Geometry: final body of the model. Coordinates: model frame, mm. A direction names the side the tool comes from. Give positions to 0.01 mm unless a question says otherwise; leave off trailing zeros. Order: outer loops, then holes, each group sorted by start corner. A loop starts at its lowest first (then second) coordinate and runs counter-clockwise, first axis right, second up. Notation, with made-up numbers: (-19.75, 3) -> (-5.75, 3) arc R19 ccw to (-5.75, 16) -> close; hole circle Ø11 at (19, 10.25). An arc over 180 degrees is marked (long way). Write item = value, one per line.
```python
from build123d import *

# Parameters (mm, degrees)
SKETCH_1_R          = 57.15
SKETCH_1_R_2        = 50.8
EXTRUDE_1_DEPTH     = 6.35
SKETCH_2_R          = 55
SKETCH_2_R_2        = 52.5
CUT_EXTRUDE_1_DEPTH = 1
CUT_EXTRUDE_START   = -1
SKETCH_3_R          = 55
SKETCH_3_R_2        = 52.5
CUT_EXTRUDE_2_DEPTH = 1
CHAMFER_1_SIZE      = 0.5


with BuildPart() as part:
    # 草图1 → 凸台-拉伸1 (new body)
    with BuildSketch(Plane(origin=(0, 0, 0), x_dir=(1, 0, 0), z_dir=(0, 1, 0))):
        with Locations(Location((0, 0, 0), (0, 0, 270))):
            Circle(SKETCH_1_R)
        with Locations(Location((0, 0, 0), (0, 0, 270))):
            Circle(SKETCH_1_R_2, mode=Mode.SUBTRACT)
    extrude(amount=EXTRUDE_1_DEPTH)

    # 草图2 → 切除-拉伸1 (cut)
    with BuildSketch(Plane(origin=(0, 6.35, 0), x_dir=(1, 0, 0), z_dir=(0, 1, 0))):
        with Locations(Location((0, 0, 0), (0, 0, 270))):
            Circle(SKETCH_2_R)
        with Locations(Location((0, 0, 0), (0, 0, 270))):
            Circle(SKETCH_2_R_2, mode=Mode.SUBTRACT)
    extrude(amount=-CUT_EXTRUDE_1_DEPTH, mode=Mode.SUBTRACT)

    # 草图3 → 切除-拉伸2 (cut)
    with BuildSketch(Plane.XZ.offset(CUT_EXTRUDE_START)):
        with Locations(Location((0, 0, 0), (0, 0, 90))):
            Circle(SKETCH_3_R)
        with Locations(Location((0, 0, 0), (0, 0, 90))):
            Circle(SKETCH_3_R_2, mode=Mode.SUBTRACT)
    extrude(amount=CUT_EXTRUDE_2_DEPTH, mode=Mode.SUBTRACT)

    # 倒角1
    chamfer_1_edges = [part.edges().sort_by_distance(p)[0] for p in [
        (0, 0, -57.15),
        (0, 6.35, -57.15),
        (0, 0, -50.8),
        (0, 6.35, -50.8),
    ]]
    chamfer(chamfer_1_edges, length=CHAMFER_1_SIZE)


solid = part.part
```
1) Line query: line 1 (X direction, y = 0.7, z = 0); line 2 (X direction, y = 6.1, z = 0); line 3 (X direction, y = 4.4, z = 0). Output: solid intervals per line, ascending. Write a range as from..to.
Check sheet entries:
line_1 = -57.15..-55, -52.5..-50.8, 50.8..52.5, 55..57.15
line_2 = -56.9..-55, -52.5..-51.05, 51.05..52.5, 55..56.9
line_3 = -57.15..-50.8, 50.8..57.15
2) First-contact query: P1, Ø1.5, axis at x = 39, y = 2.5, coming from the +Z side; P2, Ø3, axis at y = 1, z = -4, coming from the +X side; P3, Ø2, axis at y = 2.5, z = 38.5, coming from the +X side. Flat tips, straight axial feed; report the tip coordinate or a pass-through.
Check sheet entries:
P1 = 42.46
P2 = 57.1
P3 = 43.13
3) Reachability of faces 4 (the face through (-20, 5.35, 49)), 5 (the face through (55, 0, -9)), 6 (the face through (48.794, 0.507, 25.379)) from +Z, -Z, +X, -X, +Y, -Y: full face, straight path, thin tool, end or side. Return the list, or none.
Check sheet entries:
face_4 = +Y
face_5 = +Z, -Z, +X, -X, -Y
face_6 = -Y
4) Mould query, pull axis Z, two halves, no side actions, for faces 1 (the face through (-15.77, 0.507, 50.076)), 2 (the face through (2.513, 3.138, -57.095)), 3 (the face through (55, 6.35, -9)). Classes: +Z half, -Z half, draft (parallel to the pull), parting line (faces both ways), or undercut.
Check sheet entries:
face_1 = undercut
face_2 = parting line
face_3 = draft
5) Section query C-C (y = 2.5). Output: boundary loops of the cut face in (x, z).
Check sheet entries:
outline = circle Ø114.3 at (0, 0); hole circle Ø101.6 at (0, 0)
